Read the model definition and answer for the solid it produces. Units are mm, in the model's axes. A direction names the side the tool comes from. Coordinates: 2 decimals unless noted, no trailing zeros. Loops run counter-clockwise (first coordinate to the right, second up) from the corner with the lowest first, then second, coordinate; pieces in that order, holes last. Notation, with made-up numbers: M 39.25,2.5 L 48.25,2.5 A6 ccw 48.25,6.5 Z; hole C 15,-37.75 d6. An arc over 180 degrees is marked long. Put each result on its own line as item: value.
Autodesk Inventor part; units mm, degrees
ref_plane "YZ Plane" through (0, 0, 0) normal (1, 0, 0) x (0, 1, 0)
ref_plane "XZ Plane" through (0, 0, 0) normal (0, 1, 0) x (-1, 0, 0)
ref_plane "XY Plane" through (0, 0, 0) normal (0, 0, 1) x (1, 0, 0)
sketch "Sketch1" plane through (0, 0, 0) normal (0, 0, 1) x (1, 0, 0)
  line L0 (0, 0) -> (76.2, 0)
  line L1 (76.2, 0) -> (76.2, 76.2)
  line L2 (76.2, 76.2) -> (0, 76.2)
  line L3 (0, 3.175) -> (0, 0)
  line L4 (3.175, 3.175) -> (73.025, 3.175)
  line L5 (73.025, 3.175) -> (73.025, 73.025)
  line L6 (3.175, 3.175) -> (0, 3.175)
  line L7 (73.025, 73.025) -> (73.025, 76.2)
  dimension "d0" = 76.2
  dimension "d1" = 76.2
extrude "Extrusion1" add sketch "Sketch1" along normal blind 114.3
sketch "Sketch2" plane through (0, 0, 0) normal (0, -1, 0) x (1, 0, 0)
  line L0 (0, 114.3) -> (76.2, 114.3)
  line L1 (0, 0) -> (0, 114.3)
  point P0 (20.6375, 93.6625)
  dimension "d5" = 20.6375
  dimension "d6" = 20.6375
  dimension "d14" = 114.3
hole "Hole1" at (20.6375, 0, 93.6625) direction (0, 1, 0) diameter 28.575 depth 25.4 tip angle 118
sketch "Sketch3" plane through (0, 3.175, 0) normal (0, 1, 0) x (1, 0, 0)
  circle A0 centre (20.6375, -93.6625) radius 14.2875
  line L0 (0, 0) -> (0, -114.3)
  line L1 (47.625, 18.9706) -> (73.025, 18.9706) construction
  line L2 (73.025, 18.9706) -> (73.025, -101.6) construction
  line L3 (73.025, -101.6) -> (47.625, -101.6) construction
  line L4 (47.625, -101.6) -> (47.625, 18.9706) construction
  line L5 (73.025, 0) -> (73.025, -114.3) construction
  circle A1 centre (25.0952, -24.2603) radius 17.4498 construction
  dimension "d27" = 69.5452
  dimension "d28" = 25.4
  dimension "d29" = 34.8996
  dimension "d30" = 22.5298
hole "Hole2" at (25.0952, 3.175, 24.2603) direction (0, -1, 0) diameter 19.05 depth 25.4 tip angle 118
sketch "Sketch4" plane through (0, 3.175, 0) normal (0, 1, 0) x (1, 0, 0)
  line L0 (0, 0) -> (0, -114.3)
  circle A0 centre (25.0952, -24.2603) radius 25.4
  line L1 (-11.821, -6.2998) -> (92.2522, -6.2998) construction
  circle A1 centre (25.0952, -24.2603) radius 7.9375
  circle A2 centre (25.0952, -24.2603) radius 9.525
  point P0 (7.1347, -6.2998)
  point P1 (7.1347, -42.2208)
  point P2 (43.0557, -42.2208)
  point P3 (43.0557, -6.2998)
  dimension "d39" = 50.8
  dimension "d42" = 360
hole "Hole3" at (7.1347, 3.175, 6.2998) at (43.0557, 3.175, 6.2998) at (43.0557, 3.175, 42.2208) at (7.1347, 3.175, 42.2208) direction (0, -1, 0) diameter 5.1054 depth 25.4 tip angle 118
sketch "Sketch5" plane through (0, 0, 0) normal (0, 0, -1) x (-1, 0, 0)
  line L0 (-47.7073, 61.8998) -> (-105.1568, 61.8998)
  line L1 (-105.1568, 61.8998) -> (-105.1568, 87.3508)
  line L2 (-105.1568, 87.3508) -> (-47.7073, 87.3508)
  line L3 (-47.7073, 87.3508) -> (-47.7073, 61.8998)
  line L4 (-76.2, 76.2) -> (-73.025, 76.2)
  point P0 (0, 0)
  dimension "d44" = 14.3002
extrude "Extrusion2" cut sketch "Sketch5" against normal through all
sketch "Sketch6" plane through (73.025, 3.175, 0) normal (-1, 0, 0) x (0, 0, 1)
  line L0 (114.3, 58.7248) -> (0, 58.7248)
  line L1 (114.3, 58.7248) -> (114.3, 0)
  line L2 (0, 58.7248) -> (0, 0)
  point P0 (0, -3.175)
  point P1 (101.6, 46.0248)
  point P2 (88.9, 46.0248)
  point P3 (76.2, 46.0248)
  point P4 (63.5, 46.0248)
  point P5 (50.8, 46.0248)
  point P6 (38.1, 46.0248)
  point P7 (25.4, 46.0248)
  point P8 (12.7, 46.0248)
  dimension "d47" = 12.7
  dimension "d48" = 12.7
  dimension "d49" = 12.7
  dimension "d50" = 12.7
  dimension "d51" = 12.7
  dimension "d52" = 12.7
  dimension "d53" = 12.7
  dimension "d54" = 12.7
  dimension "d55" = 12.7
  dimension "d56" = 12.7
  dimension "d57" = 12.7
  dimension "d58" = 12.7
  dimension "d59" = 12.7
  dimension "d60" = 12.7
  dimension "d61" = 12.7
  dimension "d62" = 12.7
hole "Hole4" at (73.025, 49.1998, 101.6) at (73.025, 49.1998, 88.9) at (73.025, 49.1998, 76.2) at (73.025, 49.1998, 63.5) at (73.025, 49.1998, 50.8) at (73.025, 49.1998, 38.1) at (73.025, 49.1998, 25.4) at (73.025, 49.1998, 12.7) direction (1, 0, 0) diameter 4.8514 end through all
properties part number "ARM_067_NewLongShaftMount" material "Aluminum 6061"
1) Given pin 1 Ø2 at (y, z) = (52.5, 36) entering from -X (3 decimals); pin 2 Ø3 at (x, z) = (7.13, 6.3) entering from -Y; pin 3 Ø1 at (x, z) = (35, 85) entering from +Y (3 decimals), each flat-ended and moving along its own axis, determine where each tip first touches the part or whether it passes through.
Answer list:
pin 1: stops at x = 73.025
pin 2: passes through
pin 3: stops at y = 3.175
2) Find section B-B, the plane z = 88.9. Write down the section's boundary in (x, y) (1 decimal).
Answer list:
outline: M 0,0 L 7.2,0 L 7.2,3.2 L 0,3.2 Z; M 34.1,0 L 76.2,0 L 76.2,46.8 L 73,46.8 L 73,3.2 L 34.1,3.2 Z; M 73,51.6 L 76.2,51.6 L 76.2,61.9 L 73,61.9 Z
3) Which of the six approach directions +Z, -Z, +X, -X, +Y, -Y give full straight-line access (tool end or side, diameter ignored) to faces 4 (the flat face through (75, 61.9, 56)), 5 (the flat face through (73.025, 32, 56))?
Answer list:
face 4: +Z, -Z, +X, -X, +Y
face 5: +Z, -Z, -X, +Y
4) Straight lines are drawn through the part: line 1 (Y direction, x = 74.75, z = 50.8); line 2 (X direction, y = 17, z = 8) (3 decimals); line 3 (Y direction, x = 32.5, z = 7) (3 decimals). For each, find the intervals that lie inside material, in ascending order. Write a range as [from, to].
Answer list:
line 1: y = [0, 46.77], [51.63, 61.9]
line 2: x = [73.025, 76.2]
line 3: y = [0, 3.175]
5) Determine the mould class of faces 1 (the cylindrical face through (22.234, 1.565, 33.345)), 2 (the flat face through (76.2, 31, 56)), 3 (the cylindrical face through (74.63, 51.35, 13.82)) for opening direction X: released by +X, released by -X, zero draft, split by the parting line, or undercut.
Answer list:
face 1: undercut
face 2: released by +X
face 3: zero draft
6) Find section D-D, the plane z = 57.5. Write down the section's boundary in (x, y) (3 decimals).
Answer list:
outline: M 0,0 L 76.2,0 L 76.2,61.9 L 73.025,61.9 L 73.025,3.175 L 0,3.175 Z
7) Find section C-C, the plane x = 18.5. Write down the section's boundary in (y, z) (3 decimals).
Answer list:
outline: M 0,0 L 3.175,0 L 3.175,17.388 L 0,17.388 Z; M 0,31.133 L 3.175,31.133 L 3.175,79.536 L 0,79.536 Z; M 0,107.789 L 3.175,107.789 L 3.175,114.3 L 0,114.3 Z
8) Find section A-A, the plane z = 12.7. Write down the section's boundary in (x, y) (1 decimal), plus the area to 3 significant figures.
Answer list:
outline: M 0,0 L 76.2,0 L 76.2,46.8 L 73,46.8 L 73,3.2 L 0,3.2 Z; M 73,51.6 L 76.2,51.6 L 76.2,61.9 L 73,61.9 Z
area: 413 mm^2
